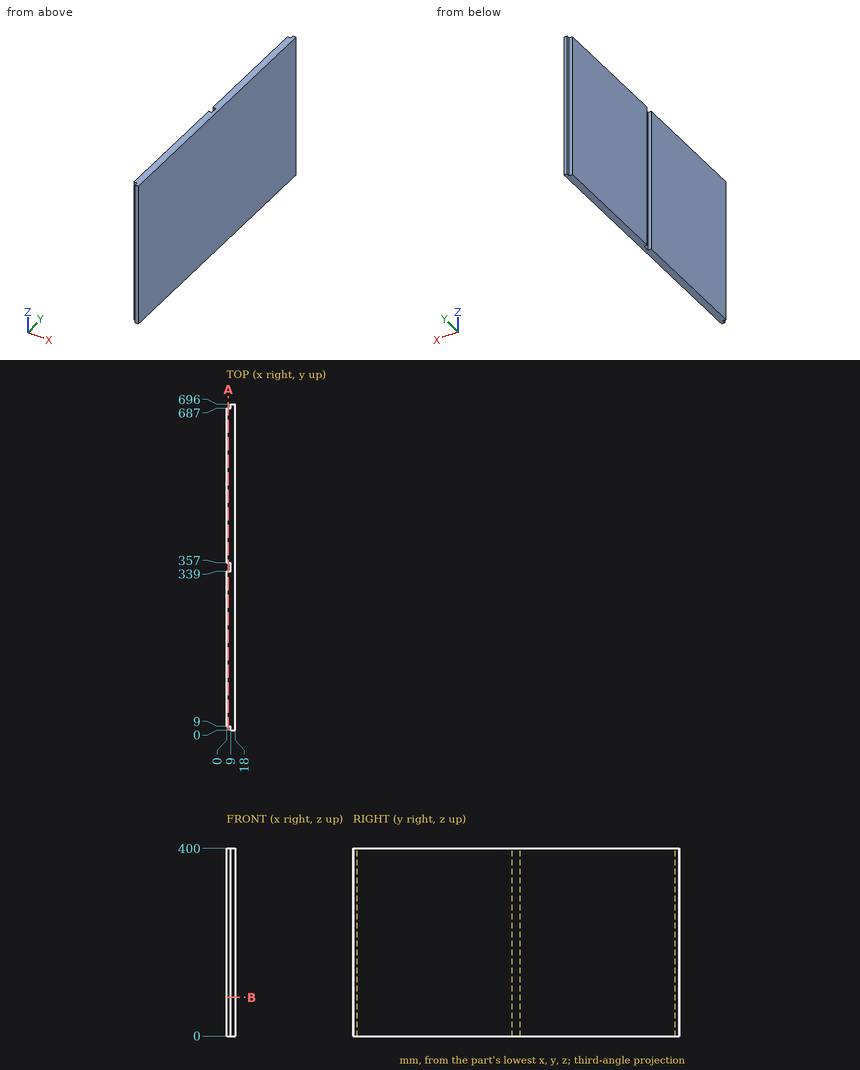
Could you check a few things on this drawing? It's one solid part, dimensions in mm from its lowest x, y, z. Coordinates: 2 decimals unless noted, no trailing zeros. Write each loop counter-clockwise with the first axis right and the second up, starting at its lowest first coordinate (ties: lowest second). Pieces come first, ordered by that corner, then holes. Notation, with made-up numbers: M 89.25,68 L 144.25,68 A10 cw 144.25,76 Z; hole C 0,-27 d4. An arc over 180 degrees is marked long. Answer as CSV lines item,"result". Start each with the question number.
Q1. Suppose I cut it at A-A, the plane x = 4. List the corners of the cut face in (y, z) for me.
Q2. Will these pins go through, and if not, where does the flat tip stop? pin 1 Ø10 at (x, z) = (3.5, 233) entering from -Y; pin 2 Ø4.5 at (y, z) = (6.5, 171.5) entering from -X; pin 3 Ø2 at (x, z) = (4.5, 99.5) entering from +Y.
Q3. I need wall thicknesses on probe 1 along Y at (x, z) = (2.25, 340.5). Which ranges of the line are inside material? Lowest first, please. Write a range as [from, to].
Q4. Suppose I cut it at B-B, the plane z = 82.5. List the corners of the cut face in (x, y) for me, then the cut area to 3 significant figures.
Entries:
1,outline,"M 9,0 L 339,0 L 339,400 L 9,400 Z; M 357,0 L 687,0 L 687,400 L 357,400 Z"
2,pin 1,"stops at y = 9"
2,pin 2,"stops at x = 9"
2,pin 3,"stops at y = 687"
3,probe 1,"y = [9, 339], [357, 687]"
4,outline,"M 0,9 L 9,9 L 9,0 L 18,0 L 18,696 L 9,696 L 9,687 L 0,687 L 0,357 L 9,357 L 9,339 L 0,339 Z"
4,area,"12,200 mm²"
